Job drawing, mm, ordinate dimensions from the low corner. One solid piece. A direction names the side the tool comes from. Round coordinates to 2 decimals unless told otherwise and drop trailing zeros. Loops run counter-clockwise (first coordinate to the right, second up) from the corner with the lowest first, then second, coordinate; pieces in that order, holes last. Notation, with made-up numbers: M 70.25,58.5 L 81.25,58.5 A18 ccw 81.25,81.5 Z; hole C 69.5,83 d7. An arc over 180 degrees is marked long. Use one line per item in the form item = value. Start each with the question number.
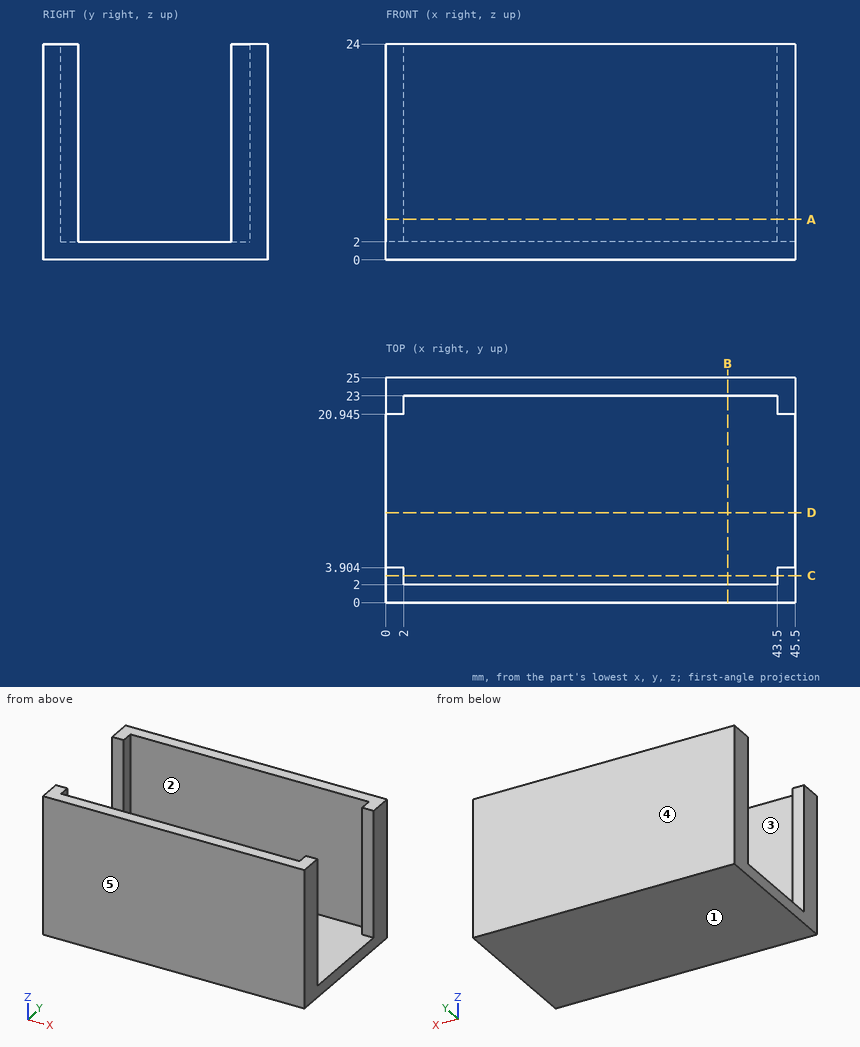
Q1. Tool access for the marked faces 1 and 2: list every direction of +Z, -Z, +X, -X, +Y, -Y with a clear straight run to the whole face (end or side of a thin tool).
Q2. Pull direction Y, two halves, no side cores. Call the marked faces 3, 4 and 5: pulls with the +Y half, pulls with the -Y half, needs draft (parallel to the pull), parting line crosses it, or undercut.
Q3. Wall check: probe 1 along Y at (x, z) = (13.5, 11.5); probe 2 along Z at (x, y) = (43, 9.75). Give the ranges that are in metal, low to high.
Q4. Saw through at A-A (z = 4.5). Give the cut face in (x, y) (1 decimal), and give its area (3 significant figures).
Q5. Saw through at B-B (x = 38). Give the cut face in (y, z), and give its area (3 significant figures).
Q6. Saw through at C-C (y = 3). Give the cut face in (x, z).
Q7. Saw through at D-D (y = 10). Give the cut face in (x, z).
Filled in:
q1.face_1 = -Z, +X, -X, +Y, -Y
q1.face_2 = +Z
q2.face_3 = undercut
q2.face_4 = pulls with the +Y half
q2.face_5 = pulls with the -Y half
q3.probe_1 = 0 to 2, 23 to 25
q3.probe_2 = 0 to 2
q4.outline = M 0,0 L 45.5,0 L 45.5,3.9 L 43.5,3.9 L 43.5,2 L 2,2 L 2,3.9 L 0,3.9 Z; M 0,20.9 L 2,20.9 L 2,23 L 43.5,23 L 43.5,20.9 L 45.5,20.9 L 45.5,25 L 0,25 Z
q4.area = 198 mm²
q5.outline = M 0,0 L 25,0 L 25,24 L 23,24 L 23,2 L 2,2 L 2,24 L 0,24 Z
q5.area = 138 mm²
q6.outline = M 0,0 L 45.5,0 L 45.5,24 L 43.5,24 L 43.5,2 L 2,2 L 2,24 L 0,24 Z
q7.outline = M 0,0 L 45.5,0 L 45.5,2 L 0,2 Z
